```python
from build123d import *

# Parameters (mm, degrees)
F0_R      = 1.75
F1_DEPTH  = 5
F3_DEPTH  = 3
F5_DEPTH  = 3
F7_DEPTH  = 17
F8_R      = 1.75
F9_DEPTH  = 17
F10_R     = 1.75
F11_DEPTH = 50


with BuildPart() as f1:
    # F0 (on Top) → F1 (new body, symmetric)
    with BuildSketch(Plane.XY):
        with BuildLine():
            ThreePointArc((7.5, -2.5), (4.571068, 4.571068), (-2.5, 7.5))
            Line((-2.5, 7.5), (-7.5, 7.5))
            Line((-7.5, 7.5), (-7.5, -7.5))
            Line((-7.5, -7.5), (7.5, -7.5))
            Line((7.5, -7.5), (7.5, -2.5))
        make_face()
        with Locations((-2.5, -2.5)):
            Circle(F0_R, mode=Mode.SUBTRACT)
    extrude(amount=F1_DEPTH, both=True)

    # F2 (on face) → F3 (join)
    with BuildSketch(Plane.XY.offset(5)):
        with BuildLine():
            Line((-7.5, 0.6), (-4.289786, 0.6))
            Line((-4.289786, 0.6), (-0.710214, 0.6))
            Line((-0.710214, 0.6), (1.079572, -2.5))
            Line((1.079572, -2.5), (-0.710214, -5.6))
            Line((-0.710214, -5.6), (-4.289786, -5.6))
            Line((-4.289786, -5.6), (-7.5, -5.6))
            Line((-7.5, -5.6), (-7.5, -7.5))
            Line((-7.5, -7.5), (7.5, -7.5))
            Line((7.5, -7.5), (7.5, -2.5))
            ThreePointArc((7.5, -2.5), (4.571068, 4.571068), (-2.5, 7.5))
            Line((-2.5, 7.5), (-7.5, 7.5))
            Line((-7.5, 7.5), (-7.5, 0.6))
        make_face()
    extrude(amount=F3_DEPTH)

    # F4 (on face) → F5 (join)
    with BuildSketch(Plane(origin=(0, 0, -5), x_dir=(1, 0, 0), z_dir=(0, 0, -1))):
        with BuildLine():
            Line((1.079572, 2.5), (-0.710214, -0.6))
            Line((-0.710214, -0.6), (-4.289786, -0.6))
            Line((-4.289786, -0.6), (-7.5, -0.6))
            Line((-7.5, -0.6), (-7.5, -7.5))
            Line((-7.5, -7.5), (-2.5, -7.5))
            ThreePointArc((-2.5, -7.5), (4.571068, -4.571068), (7.5, 2.5))
            Line((7.5, 2.5), (7.5, 7.5))
            Line((7.5, 7.5), (-7.5, 7.5))
            Line((-7.5, 7.5), (-7.5, 5.6))
            Line((-7.5, 5.6), (-4.289786, 5.6))
            Line((-4.289786, 5.6), (-0.710214, 5.6))
            Line((-0.710214, 5.6), (1.079572, 2.5))
        make_face()
    extrude(amount=F5_DEPTH)

    # F6 (on face) → F7 (join)
    with BuildSketch(Plane.XY.offset(8)):
        with BuildLine():
            Line((-7.5, 7.5), (-7.5, -7.5))
            Line((-7.5, -7.5), (7.5, -7.5))
            Line((7.5, -7.5), (7.5, -2.5))
            ThreePointArc((7.5, -2.5), (4.571068, 4.571068), (-2.5, 7.5))
            Line((-2.5, 7.5), (-7.5, 7.5))
        make_face()
    extrude(amount=F7_DEPTH)

    # F8 (on face) → F9 (join)
    with BuildSketch(Plane(origin=(0, 0, -8), x_dir=(1, 0, 0), z_dir=(0, 0, -1))):
        with BuildLine():
            Line((7.5, 7.5), (-7.5, 7.5))
            Line((-7.5, 7.5), (-7.5, -7.5))
            Line((-7.5, -7.5), (-2.5, -7.5))
            ThreePointArc((-2.5, -7.5), (4.571068, -4.571068), (7.5, 2.5))
            Line((7.5, 2.5), (7.5, 7.5))
        make_face()
        with Locations((-2.5, 2.5)):
            Circle(F8_R, mode=Mode.SUBTRACT)
    extrude(amount=F9_DEPTH)

    # F10 (on face) → F11 (cut)
    with BuildSketch(Plane.XY.offset(25)):
        with Locations((-2.5, -2.5)):
            Circle(F10_R)
    extrude(amount=-F11_DEPTH, mode=Mode.SUBTRACT)


solid = f1.part
```
CAD build for the part. Positions are in the model's coordinates, mm. A direction names the side the tool comes from. Round coordinates to 2 decimals unless told otherwise and drop trailing zeros. Order: outer loops, then holes, each group sorted by start corner. A loop starts at its lowest first (then second) coordinate and runs counter-clockwise, first axis right, second up. Notation, with made-up numbers: (31, 41.5) - (90, 41.5) arc R33 ccw to (90, 70.5) - close; hole circle Ø2 at (73.5, 10.5). An arc over 180 degrees is marked (long way). Answer in a Markdown table with one row per item. Add a question column.
(1) 3-axis set-ups, long thin cutter, end or side, ignore diameter. For faces 3 (the face through (-5, -2, 8)), 4 (the face through (-7.5, 0, 0)): which of +Z, -Z, +X, -X, +Y, -Y reach the whole face in a straight line?
(2) Band-saw the part on C-C on y = 4. List the corners of the cut face in (x, z), and give its area (3 significant figures).
(3) Band-saw the part on B-B on z = 9.5. List the corners of the cut face in (x, y), and give its area (3 significant figures).
(4) Drop flat-ended pins along their axis: pin 1 Ø4 at (x, z) = (2.5, 9) entering from +Y; pin 2 Ø3 at (y, z) = (3.5, -9.5) entering from +X; pin 3 Ø3 at (x, y) = (-2.5, -2.5) entering from -Z; pin 4 Ø1.5 at (y, z) = (5.5, -19) entering from +X. Give the stop position or say it passes through.
(5) Mould opens along Y. For faces 1 (the face through (7.5, -5, 0)), 2 (the face through (0.197, -4.028, 6.479)) say: +Y half, -Y half, draft (parallel to the pull), parting line (faces both ways), or undercut.
(6) Probe L1, parallel to Y at x = -2.5, z = -13; L2, parallel to Z at x = -6.25, y = -1.5. List the from-to ranges inside material, lowest first. Write a range as [from, to].
(7) Band-saw the part on A-A on y = -3. List the corners of the cut face in (x, z).
(8) Band-saw the part on D-D on x = 2.75. List the corners of the cut face in (y, z).
Data:
| question | item | result |
|---|---|---|
| 1 | face 3 | -X |
| 1 | face 4 | +Z, -Z, -X, +Y, -Y |
| 2 | outline | (-7.5, -25) - (5.1, -25) - (5.1, 25) - (-7.5, 25) - close |
| 2 | area | 630 mm^2 |
| 3 | outline | (-7.5, -7.5) - (7.5, -7.5) - (7.5, -2.5) arc R10 ccw to (-2.5, 7.5) - (-7.5, 7.5) - close; hole circle Ø3.5 at (-2.5, -2.5) |
| 3 | area | 194 mm^2 |
| 4 | pin 1 | stops at y = 7.04 |
| 4 | pin 2 | stops at x = 6.43 |
| 4 | pin 3 | passes through |
| 4 | pin 4 | stops at x = 4.39 |
| 5 | face 1 | draft |
| 5 | face 2 | undercut |
| 6 | L1 | y = [-7.5, -4.25], [-0.75, 7.5] |
| 6 | L2 | z = [-25, -8], [-5, 5], [8, 25] |
| 7 | outline | (-7.5, -25) - (-4.18, -25) - (-4.18, -8) - (-7.5, -8) - close; (-7.5, -5) - (-4.18, -5) - (-4.18, 5) - (-7.5, 5) - close; (-7.5, 8) - (-4.18, 8) - (-4.18, 25) - (-7.5, 25) - close; (-0.82, -25) - (7.5, -25) - (7.5, 25) - (-0.82, 25) - (-0.82, 8) - (0.79, 8) - (0.79, 5) - (-0.82, 5) - (-0.82, -5) - (0.79, -5) - (0.79, -8) - (-0.82, -8) - close |
| 8 | outline | (-7.5, -25) - (6.01, -25) - (6.01, 25) - (-7.5, 25) - close |
